```python
from build123d import *

# Parameters (mm, degrees)
SKETCH2_R                = 3.9751
BOSS_EXTRUDE1_DEPTH      = 5.6
M4X0_7_TAPPED_HOLE1_D    = 3.3
SKETCH7_R                = 2.75
SKETCH7_R_2              = 1.65
BOSS_EXTRUDE2_DEPTH      = 0.675
BOSS_EXTRUDE2_DEPTH_BACK = 11.875
SKETCH9_R                = 3.9751
SKETCH9_R_2              = 2.75
CUT_EXTRUDE1_DEPTH       = 0.2
SKETCH10_R               = 3.9751
SKETCH10_R_2             = 2.75
CUT_EXTRUDE3_DEPTH       = 0.2


with BuildPart() as part:
    # Sketch2 → Boss-Extrude1 (new, symmetric)
    with BuildSketch(Plane(origin=(0, 0, 0), x_dir=(1, 0, 0), z_dir=(0, 1, 0))):
        with Locations(Location((0, 0, 0), (0, 0, 270))):
            Circle(SKETCH2_R)
    extrude(amount=BOSS_EXTRUDE1_DEPTH, both=True)

    # M4x0.7 Tapped Hole1 (through all)
    with Locations(Plane(origin=(0, 5.6, 0), x_dir=(1, 0, 0), z_dir=(0, 1, 0))):
        with Locations((0, 0)):
            Hole(M4X0_7_TAPPED_HOLE1_D / 2)

    # Sketch7 → Boss-Extrude2 (add, two sides)
    with BuildSketch(Plane(origin=(0, 5.6, 0), x_dir=(1, 0, 0), z_dir=(0, 1, 0))) as boss_extrude2_sk:
        with Locations(Location((0, 0, 0), (0, 0, 270))):
            Circle(SKETCH7_R)
        with Locations(Location((0, 0, 0), (0, 0, 270))):
            Circle(SKETCH7_R_2, mode=Mode.SUBTRACT)
    extrude(amount=BOSS_EXTRUDE2_DEPTH)
    extrude(boss_extrude2_sk.sketch, amount=-BOSS_EXTRUDE2_DEPTH_BACK)

    # Sketch9 → Cut-Extrude1 (cut)
    with BuildSketch(Plane(origin=(0, 5.6, 0), x_dir=(1, 0, 0), z_dir=(0, 1, 0))):
        with Locations(Location((0, 0, 0), (0, 0, 270))):
            Circle(SKETCH9_R)
        with Locations(Location((0, 0, 0), (0, 0, 270))):
            Circle(SKETCH9_R_2, mode=Mode.SUBTRACT)
    extrude(amount=-CUT_EXTRUDE1_DEPTH, mode=Mode.SUBTRACT)

    # Sketch10 → Cut-Extrude3 (cut)
    with BuildSketch(Plane.XZ.offset(5.6)):
        with Locations(Location((0, 0, 0), (0, 0, 270))):
            Circle(SKETCH10_R)
        with Locations(Location((0, 0, 0), (0, 0, 90))):
            Circle(SKETCH10_R_2, mode=Mode.SUBTRACT)
    extrude(amount=-CUT_EXTRUDE3_DEPTH, mode=Mode.SUBTRACT)


solid = part.part
```
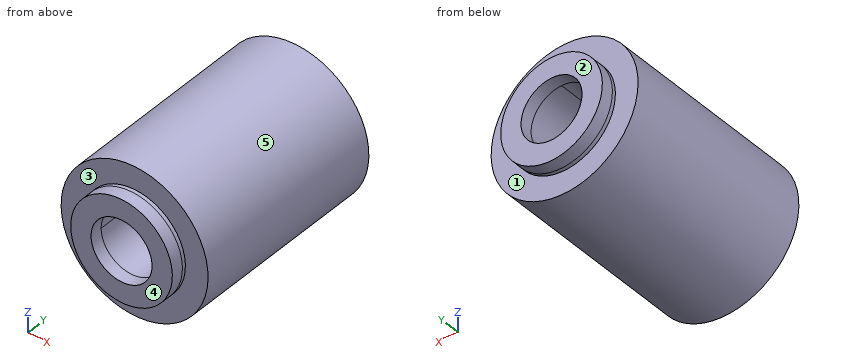
CAD build for the part. Positions are in the model's coordinates, mm. Face numbers are marked on the shaded views. A direction names the side the tool comes from. Coordinates: 2 decimals unless noted, no trailing zeros. Write each loop counter-clockwise with the first axis right and the second up, starting at its lowest first coordinate (ties: lowest second). Pieces come first, ordered by that corner, then holes. Notation, with made-up numbers: (57, -2.5) -> (80, -2.5) arc R24 ccw to (80, 14.5) -> close; hole circle Ø1 at (28, -27.75). An arc over 180 degrees is marked (long way). Return JSON: item names as keys, results as strings. Group by question number.
Q1. Pull direction Z, two halves, no side cores. Call the marked faces 4 and 5: released by +Z, released by -Z, zero draft, split by the parting line, or undercut.
Q2. Drill centre lines: line 1 (X direction, y = 5.95, z = 0); line 2 (Z direction, x = 0, y = 1.25); line 3 (Z direction, x = 1.25, y = -4). Where is each one in solid material? Low to high.
Q3. Cut at C-C, the plane x = -2.5. Give the cut face in (y, z) (3 decimals), then the cut area to 3 significant figures.
Q4. Flat gauge pin, fed straight in: pin 1 (1 mm diameter, centred on y = 2, z = 3, fed in from -X). Where does the tip first touch, or does it go through?
Q5. Which spindle directions (+Z, -Z, +X, -X, +Y, -Y) get a long thin tool onto all of the face, cutting with end or side? Do the marked faces 1, 2 and 3. Say none if no direction does.
Q6. Cut at D-D, the plane z = -3. Give the cut face in (x, y).
Q7. Cut at B-B, the plane y = -5. Give the cut face in (x, z).
Q8. Cut at A-A, the plane x = 0.5. Give the cut face in (y, z) (3 decimals), then the cut area to 3 significant figures.
Returned:
{
 "1": {"face 4": "zero draft", "face 5": "split by the parting line"},
 "2": {"line 1": "x = -2.75 to -1.65, 1.65 to 2.75", "line 2": "z = -3.98 to -1.65, 1.65 to 3.98", "line 3": "z = -3.77 to -1.08, 1.08 to 3.77"},
 "3": {"outline": "(-6.275, -1.146) -> (-5.4, -1.146) -> (-5.4, -3.091) -> (5.4, -3.091) -> (5.4, -1.146) -> (6.275, -1.146) -> (6.275, 1.146) -> (5.4, 1.146) -> (5.4, 3.091) -> (-5.4, 3.091) -> (-5.4, 1.146) -> (-6.275, 1.146) -> close", "area": "70.8 mm2"},
 "4": {"pin 1": "stops at x = -3.09"},
 "5": {"face 1": "+Y", "face 2": "+Z, -Z, +X, -X, +Y", "face 3": "-Y"},
 "6": {"outline": "(-2.61, -5.4) -> (2.61, -5.4) -> (2.61, 5.4) -> (-2.61, 5.4) -> close"},
 "7": {"outline": "circle Ø7.95 at (0, 0); hole circle Ø3.3 at (0, 0)"},
 "8": {"outline": "(-6.275, -2.704) -> (-5.4, -2.704) -> (-5.4, -3.944) -> (5.4, -3.944) -> (5.4, -2.704) -> (6.275, -2.704) -> (6.275, -1.572) -> (-6.275, -1.572) -> close; (-6.275, 1.572) -> (6.275, 1.572) -> (6.275, 2.704) -> (5.4, 2.704) -> (5.4, 3.944) -> (-5.4, 3.944) -> (-5.4, 2.704) -> (-6.275, 2.704) -> close", "area": "55.2 mm2"}
}
